Check sheet for the modelled part. Datum: model origin and axes. Units: mm. Face numbers are marked on the shaded views. A direction names the side the tool comes from. Round coordinates to 2 decimals unless told otherwise and drop trailing zeros. Write each loop counter-clockwise with the first axis right and the second up, starting at its lowest first coordinate (ties: lowest second). Pieces come first, ordered by that corner, then holes. Notation, with made-up numbers: M -32.5,18.5 L -25.5,18.5 A20 cw -25.5,23.5 Z; hole C -30,34.5 d8. An arc over 180 degrees is marked long. Put each result on its own line as item: value.
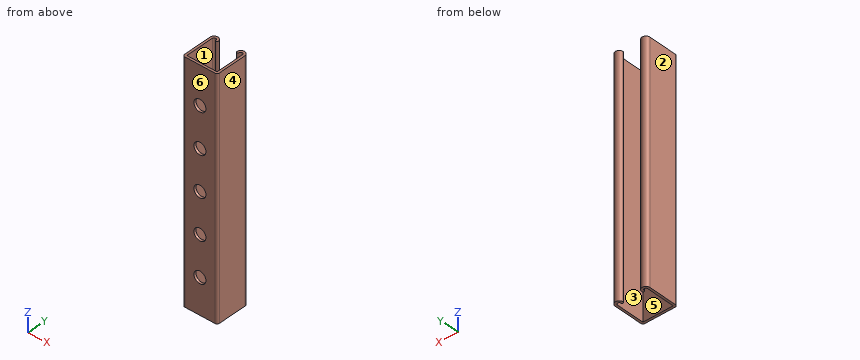
```python
from build123d import *

# Parameters (mm, degrees)
BOSS_EXTRUDE1_DEPTH = 278.384
SKETCH2_R           = 7.112
CUT_EXTRUDE1_DEPTH  = 285.075569203
LPATTERN1_COUNT     = 5
LPATTERN1_PITCH     = 47.752


with BuildPart() as part:
    # Sketch1 → Boss-Extrude1 (new body)
    with BuildSketch(Plane.XY):
        with BuildLine():
            Line((0, 0), (35.98, 0))
            ThreePointArc((35.98, 0), (37.883814298, 0.788585702), (38.6724, 2.6924))
            Line((38.6724, 2.6924), (38.6724, 36.5252))
            ThreePointArc((38.6724, 36.5252), (33.8972, 41.3004), (29.122, 36.5252))
            ThreePointArc((29.122, 36.5252), (30.4682, 35.179), (31.8144, 36.5252))
            ThreePointArc((31.8144, 36.5252), (33.8972, 38.608), (35.98, 36.5252))
            Line((35.98, 36.5252), (35.98, 2.6924))
            Line((35.98, 2.6924), (0, 2.6924))
            Line((0, 2.6924), (0, 36.5252))
            ThreePointArc((0, 36.5252), (2.0828, 38.608), (4.1656, 36.5252))
            ThreePointArc((4.1656, 36.5252), (5.5118, 35.179), (6.858, 36.5252))
            ThreePointArc((6.858, 36.5252), (2.0828, 41.3004), (-2.6924, 36.5252))
            Line((-2.6924, 36.5252), (-2.6924, 2.6924))
            ThreePointArc((-2.6924, 2.6924), (-1.903814298, 0.788585702), (0, 0))
        make_face()
    extrude(amount=BOSS_EXTRUDE1_DEPTH)

    # Sketch2 → Cut-Extrude1 (cut, through all)
    with BuildSketch(Plane(origin=(0, 0, 0), x_dir=(-1, 0, 0), z_dir=(0, -1, 0))):
        with Locations(Location((-17.99, -42.164, 0), (0, 0, 90))):
            Circle(SKETCH2_R)
    cut_extrude1 = extrude(amount=-CUT_EXTRUDE1_DEPTH, mode=Mode.SUBTRACT)

    # LPattern1: Cut-Extrude1 ×5
    with Locations(*[(0, 0, i * LPATTERN1_PITCH) for i in range(1, LPATTERN1_COUNT)]):
        add(cut_extrude1, mode=Mode.SUBTRACT)


solid = part.part
```
1. Access from +Z, -Z, +X, -X, +Y, -Y to the whole of each face (thin tool, end or side, straight path). Record for the marked faces 1 and 2.
Computed values:
face 1: +Z, -Z
face 2: +Z, -Z, -X, +Y, -Y
2. Cross-section at B-B (x = 17.99). Enter the section's corners in (y, z).
Computed values:
outline: M 0,0 L 2.69,0 L 2.69,35.05 L 0,35.05 Z; M 0,49.28 L 2.69,49.28 L 2.69,82.8 L 0,82.8 Z; M 0,97.03 L 2.69,97.03 L 2.69,130.56 L 0,130.56 Z; M 0,144.78 L 2.69,144.78 L 2.69,178.31 L 0,178.31 Z; M 0,192.53 L 2.69,192.53 L 2.69,226.06 L 0,226.06 Z; M 0,240.28 L 2.69,240.28 L 2.69,278.38 L 0,278.38 Z
3. Cross-section at A-A (y = 30). Enter the section's corners in (x, z).
Computed values:
outline: M -2.69,0 L 0,0 L 0,278.38 L -2.69,278.38 Z; M 35.98,0 L 38.67,0 L 38.67,278.38 L 35.98,278.38 Z
4. Depth check by flat-ended pin: pin 1 Ø5 at (x, z) = (26, 118.5) entering from +Y; pin 2 Ø18 at (x, z) = (24, 207) entering from +Y; pin 3 Ø23 at (x, z) = (17.99, 137.668) entering from +Y. Enter the tip coordinate at first touch or a pass-through.
Computed values:
pin 1: stops at y = 2.69
pin 2: stops at y = 41.22
pin 3: stops at y = 38.36
5. Release check for a two-part mould opening along Y. For the marked faces 3, 4, 5 and 6 record: +Y half, -Y half, draft (parallel to the pull), parting line (faces both ways), or undercut.
Computed values:
face 3: undercut
face 4: draft
face 5: undercut
face 6: -Y half
6. Scan lines: probe 1 along X at (y, z) = (22, 157); probe 2 along X at (y, z) = (36.5, 155); probe 3 along Z at (x, y) = (17, 1). Record each from-to range of solid material in increasing order.
Computed values:
probe 1: x = -2.69 to 0, 35.98 to 38.67
probe 2: x = -2.69 to 0, 4.17 to 6.86, 29.12 to 31.81, 35.98 to 38.67
probe 3: z = 0 to 35.12, 49.21 to 82.87, 96.96 to 130.63, 144.71 to 178.38, 192.46 to 226.13, 240.21 to 278.38
